Check sheet for the modelled part. Datum: model origin and axes. Units: mm. Face numbers are marked on the shaded views. A direction names the side the tool comes from. Give positions to 0.01 mm unless a question says otherwise; leave off trailing zeros. Order: outer loops, then holes, each group sorted by start corner. A loop starts at its lowest first (then second) coordinate and runs counter-clockwise, first axis right, second up.
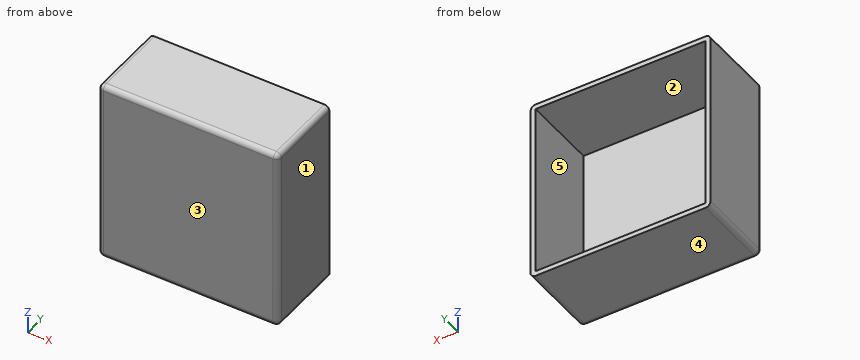
from build123d import *

# Parameters (mm, degrees)
SKETCH_1_W          = 36
SKETCH_1_H          = 37
EXTRUDE_2_DEPTH     = 16
SKETCH_2_W          = 34
SKETCH_2_H          = 35
CUT_EXTRUDE_1_DEPTH = 15
FILLET_1_R          = 1


with BuildPart() as part:
    # ｽｹｯﾁ1 → ﾎﾞｽ - 押し出し2 (new body)
    with BuildSketch(Plane(origin=(0, 0, 0), x_dir=(1, 0, 0), z_dir=(0, 1, 0))):
        with Locations((-2.682211452, 11.454993769)):
            Rectangle(SKETCH_1_W, SKETCH_1_H)
    extrude(amount=EXTRUDE_2_DEPTH)

    # ｽｹｯﾁ2 → ｶｯﾄ - 押し出し1 (cut)
    with BuildSketch(Plane(origin=(0, 16, 0), x_dir=(1, 0, 0), z_dir=(0, 1, 0))):
        with Locations((-2.682211452, 11.454993769)):
            Rectangle(SKETCH_2_W, SKETCH_2_H)
    extrude(amount=-CUT_EXTRUDE_1_DEPTH, mode=Mode.SUBTRACT)

    # ﾌｨﾚｯﾄ1
    fillet_1_edges = [part.edges().sort_by_distance(p)[0] for p in [
        (-2.682211452, 0, -29.954993769),
        (15.317788548, 0, -11.454993769),
        (-2.682211452, 0, 7.045006231),
        (-20.682211452, 0, -11.454993769),
        (-20.682211452, 8, -29.954993769),
        (15.317788548, 8, -29.954993769),
        (15.317788548, 8, 7.045006231),
        (-20.682211452, 8, 7.045006231),
    ]]
    fillet(fillet_1_edges, radius=FILLET_1_R)


solid = part.part
1) Section check B-B, the plane y = 4. Record the cut outline in (x, z) (3 decimals), then the cut area to 3 significant figures.
Recorded:
outline: (-20.682, -28.955) arc R1 ccw to (-19.682, -29.955) - (14.318, -29.955) arc R1 ccw to (15.318, -28.955) - (15.318, 6.045) arc R1 ccw to (14.318, 7.045) - (-19.682, 7.045) arc R1 ccw to (-20.682, 6.045) - close; hole (-19.682, -28.955) - (14.318, -28.955) - (14.318, 6.045) - (-19.682, 6.045) - close
area: 141 mm2
2) Material ranges on L1, parallel to X at y = 5.75, z = -11.5; L2, parallel to Z at x = -17.5, y = 11.5 (3 decimals); L3, parallel to Y at x = 3.5, z = -16, recorded low to high.
Recorded:
L1: x = -20.68 to -19.68, 14.32 to 15.32
L2: z = -29.955 to -28.955, 6.045 to 7.045
L3: y = 0 to 1
3) Draft check along Z on the marked faces 3, 4 and 5. Enter one of: +Z half, -Z half, draft (parallel to the pull), parting line (faces both ways), or undercut.
Recorded:
face 3: draft
face 4: -Z half
face 5: undercut
4) Depth check by flat-ended pin: pin 1 Ø6 at (x, z) = (4.5, -23.5) entering from +Y. Enter the tip coordinate at first touch or a pass-through.
Recorded:
pin 1: stops at y = 1
5) Section check A-A, the plane x = 1. Record the cut outline in (y, z) (3 decimals).
Recorded:
outline: (0, -28.955) arc R1 ccw to (1, -29.955) - (16, -29.955) - (16, -28.955) - (1, -28.955) - (1, 6.045) - (16, 6.045) - (16, 7.045) - (1, 7.045) arc R1 ccw to (0, 6.045) - close
6) Set-up check for the marked faces 1 and 2: record each of +Z, -Z, +X, -X, +Y, -Y from which the full face is reachable in a straight line by a thin tool's end or side.
Recorded:
face 1: +Z, -Z, +X, +Y, -Y
face 2: +Y
7) Section check C-C, the plane z = -13. Record the cut outline in (x, y).
Recorded:
outline: (-20.68, 1) arc R1 ccw to (-19.68, 0) - (14.32, 0) arc R1 ccw to (15.32, 1) - (15.32, 16) - (14.32, 16) - (14.32, 1) - (-19.68, 1) - (-19.68, 16) - (-20.68, 16) - close
